from build123d import *

# Parameters (mm, degrees)
ESQUISSE1_W             = 50
ESQUISSE1_H             = 35
BOSS_EXTRU_1_DEPTH      = 3
ESQUISSE2_R             = 1.5
ENL_V_MAT_EXTRU_1_DEPTH = 3
CONG_1_R                = 1


with BuildPart() as part:
    # Esquisse1 → Boss.-Extru.1 (new body)
    with BuildSketch(Plane.XY):
        with Locations((25, 17.5)):
            Rectangle(ESQUISSE1_W, ESQUISSE1_H)
    extrude(amount=BOSS_EXTRU_1_DEPTH)

    # Esquisse2 → Enlèv. mat.-Extru.1 (cut)
    with BuildSketch(Plane.XY.offset(3)):
        with Locations((5, 32.5)):
            Circle(ESQUISSE2_R)
        with Locations((15, 32.5)):
            Circle(ESQUISSE2_R)
        with Locations((25, 32.5)):
            Circle(ESQUISSE2_R)
        with Locations((35, 32.5)):
            Circle(ESQUISSE2_R)
        with Locations((45, 32.5)):
            Circle(ESQUISSE2_R)
        with Locations((15, 22.5)):
            Circle(ESQUISSE2_R)
        with Locations((25, 22.5)):
            Circle(ESQUISSE2_R)
        with Locations((35, 22.5)):
            Circle(ESQUISSE2_R)
        with Locations((45, 22.5)):
            Circle(ESQUISSE2_R)
        with Locations((15, 12.5)):
            Circle(ESQUISSE2_R)
        with Locations((25, 12.5)):
            Circle(ESQUISSE2_R)
        with Locations((35, 12.5)):
            Circle(ESQUISSE2_R)
        with Locations((45, 12.5)):
            Circle(ESQUISSE2_R)
        with Locations((15, 2.5)):
            Circle(ESQUISSE2_R)
        with Locations((25, 2.5)):
            Circle(ESQUISSE2_R)
        with Locations((35, 2.5)):
            Circle(ESQUISSE2_R)
        with Locations((45, 2.5)):
            Circle(ESQUISSE2_R)
        with Locations((5, 22.5)):
            Circle(ESQUISSE2_R)
        with Locations((5, 12.5)):
            Circle(ESQUISSE2_R)
        with Locations((5, 2.5)):
            Circle(ESQUISSE2_R)
    extrude(amount=-ENL_V_MAT_EXTRU_1_DEPTH, mode=Mode.SUBTRACT)

    # Congé1
    cong_1_edges = [part.edges().sort_by_distance(p)[0] for p in [
        (0, 35, 1.5),
        (50, 35, 1.5),
        (50, 0, 1.5),
        (0, 0, 1.5),
    ]]
    fillet(cong_1_edges, radius=CONG_1_R)


solid = part.part
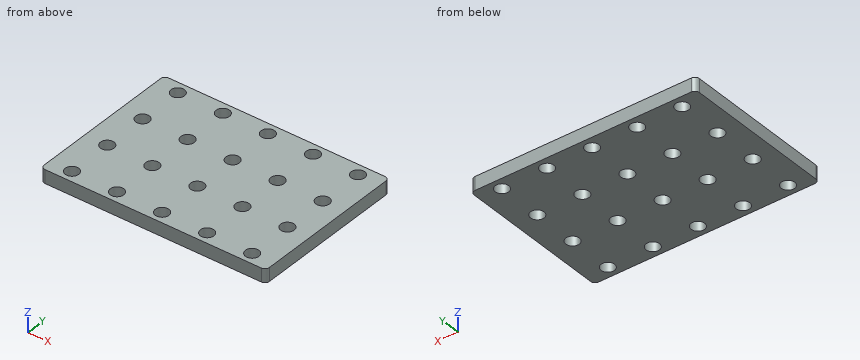
Work out the finished part from the listing and answer in its coordinate system (mm). Give positions to 0.01 mm unless a question says otherwise; leave off trailing zeros. Loops run counter-clockwise (first coordinate to the right, second up) from the corner with the lowest first, then second, coordinate; pieces in that order, holes last. Notation, with made-up numbers: (40.25, -0.75) -> (56.25, -0.75) arc R27 ccw to (56.25, 29.25) -> close; hole circle Ø8 at (54, -14.5). An arc over 180 degrees is marked (long way). Use a Markdown table: item, result. Add a question column.
1) The part is cut by section D-D, the plane x = 6. Determine the outline of the cut face in (y, z).
2) This flat-tipped pin is pushed along its axis until it touches: P1, Ø5, axis at x = 25, y = 2.5, coming from the -Z side. Where does it stop, or does it pass through?
3) The part is cut by section A-A, the plane z = 1.5. Count the separate pieces of the cut face and the enclosed holes in it, plus the area to 3 significant figures.
4) The part is cut by section B-B, the plane y = 32.5. Determine the outline of the cut face in (x, z), plus the area to 3 significant figures.
5) Consider line 1 along Y through (x, z) = (45, 2.35); line 2 along X through (y, z) = (23, 0.9); line 3 along X through (y, z) = (13.5, 0.1). Determine where each line is inside the solid, lowest interval first.
6) The part is cut by section C-C, the plane x = 25. Determine the outline of the cut face in (y, z).
Reported:
| question | item | result |
|---|---|---|
| 1 | outline | (0, 0) -> (1.38, 0) -> (1.38, 3) -> (0, 3) -> close; (3.62, 0) -> (11.38, 0) -> (11.38, 3) -> (3.62, 3) -> close; (13.62, 0) -> (21.38, 0) -> (21.38, 3) -> (13.62, 3) -> close; (23.62, 0) -> (31.38, 0) -> (31.38, 3) -> (23.62, 3) -> close; (33.62, 0) -> (35, 0) -> (35, 3) -> (33.62, 3) -> close |
| 2 | P1 | stops at z = 0 |
| 3 | separate pieces | 1 |
| 3 | enclosed holes | 20 |
| 3 | area | 1,610 mm^2 |
| 4 | outline | (0, 0) -> (3.5, 0) -> (3.5, 3) -> (0, 3) -> close; (6.5, 0) -> (13.5, 0) -> (13.5, 3) -> (6.5, 3) -> close; (16.5, 0) -> (23.5, 0) -> (23.5, 3) -> (16.5, 3) -> close; (26.5, 0) -> (33.5, 0) -> (33.5, 3) -> (26.5, 3) -> close; (36.5, 0) -> (43.5, 0) -> (43.5, 3) -> (36.5, 3) -> close; (46.5, 0) -> (50, 0) -> (50, 3) -> (46.5, 3) -> close |
| 4 | area | 105 mm^2 |
| 5 | line 1 | y = 0 to 1, 4 to 11, 14 to 21, 24 to 31, 34 to 35 |
| 5 | line 2 | x = 0 to 3.59, 6.41 to 13.59, 16.41 to 23.59, 26.41 to 33.59, 36.41 to 43.59, 46.41 to 50 |
| 5 | line 3 | x = 0 to 3.88, 6.12 to 13.88, 16.12 to 23.88, 26.12 to 33.88, 36.12 to 43.88, 46.12 to 50 |
| 6 | outline | (0, 0) -> (1, 0) -> (1, 3) -> (0, 3) -> close; (4, 0) -> (11, 0) -> (11, 3) -> (4, 3) -> close; (14, 0) -> (21, 0) -> (21, 3) -> (14, 3) -> close; (24, 0) -> (31, 0) -> (31, 3) -> (24, 3) -> close; (34, 0) -> (35, 0) -> (35, 3) -> (34, 3) -> close |
